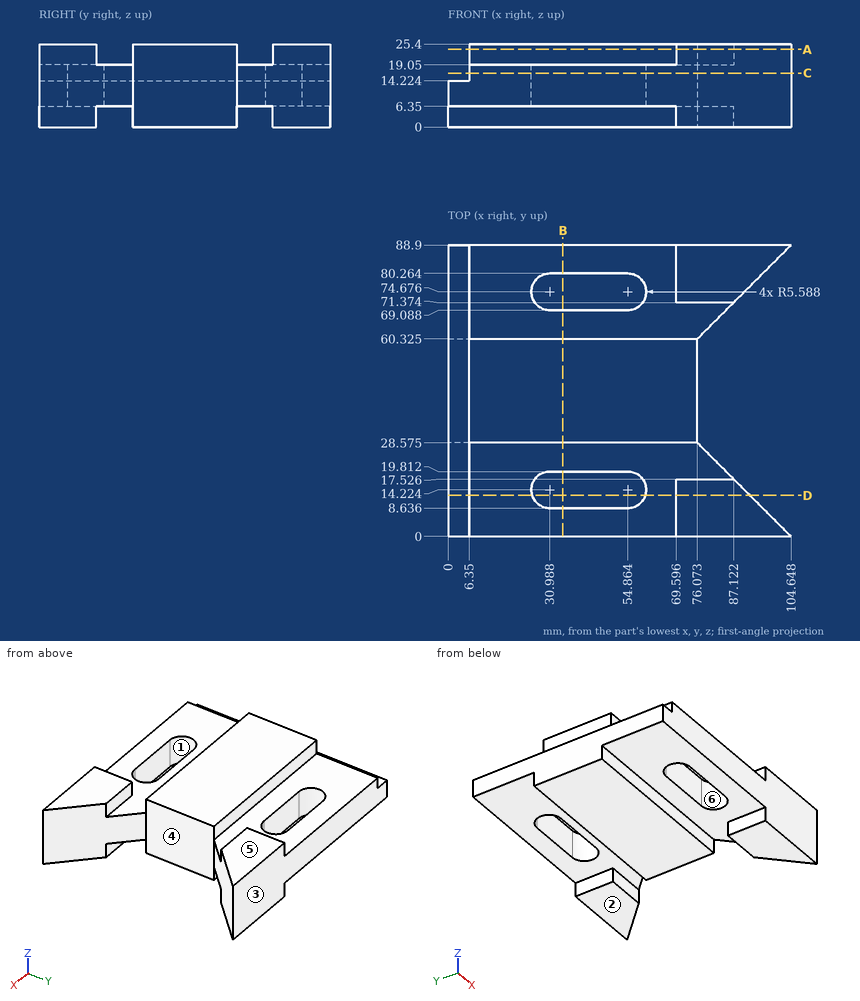
Check sheet for the drawn part. Datum: minimum x, y, z corner. Units: mm. A direction names the side the tool comes from. Round coordinates to 2 decimals unless told otherwise and drop trailing zeros. Loops run counter-clockwise (first coordinate to the right, second up) from the corner with the lowest first, then second, coordinate; pieces in that order, holes last. Notation, with made-up numbers: (-32.75, -36.5) - (-20.75, -36.5) arc R20 ccw to (-20.75, 2.5) - close; hole circle Ø9 at (70.25, 48.25). An arc over 180 degrees is marked (long way). Write item = value, one per line. Start each with the question number.
1. Section check D-D on y = 12.5. Enter the section's corners in (x, z).
2. Section check B-B on x = 35. Enter the section's corners in (y, z) (3 decimals), then the cut area to 3 significant figures.
3. Section check C-C on z = 16.5. Enter the section's corners in (x, y) (3 decimals), then the cut area to 3 significant figures.
4. Set-up check for the marked faces 4, 5 and 6: record each of +Z, -Z, +X, -X, +Y, -Y from which the full face is reachable in a straight line by a thin tool's end or side.
5. Mould release check, pull along Y, two halves, no side actions. Record for the marked faces 1, 2 and 3: released by +Y, released by -Y, zero draft, split by the parting line, or undercut.
6. Section check A-A on z = 23.75. Enter the section's corners in (x, y) (3 decimals).
7. Depth check by flat-ended pin: pin 1 (5 mm diameter, centred on x = 56, y = 71, fed in from -Z); pin 2 (3 mm diameter, centred on x = 75.5, y = 65, fed in from +Z); pin 3 (1.9 mm diameter, centred on x = 75.5, z = 4, fed in from -Y); pin 4 (3.5 mm diameter, centred on y = 44, z = 17, fed in from -X). Enter the tip coordinate at first touch or a pass-through.
8. Thickness scan on line 1 (Y direction, x = 35.5, z = 8.25); line 2 (Y direction, x = 73.5, z = 21.5) (3 decimals); line 3 (Z direction, x = 34.5, y = 85). Record the ranges inside material, lowest first.
Working result:
q1.outline = (0, 6.35) - (25.67, 6.35) - (25.67, 19.05) - (6.35, 19.05) - (6.35, 14.22) - (0, 14.22) - close; (60.18, 6.35) - (69.6, 6.35) - (69.6, 0) - (92.15, 0) - (92.15, 25.4) - (69.6, 25.4) - (69.6, 19.05) - (60.18, 19.05) - close
q2.outline = (0, 6.35) - (8.636, 6.35) - (8.636, 19.05) - (0, 19.05) - close; (19.812, 6.35) - (28.575, 6.35) - (28.575, 0) - (60.325, 0) - (60.325, 6.35) - (69.088, 6.35) - (69.088, 19.05) - (60.325, 19.05) - (60.325, 25.4) - (28.575, 25.4) - (28.575, 19.05) - (19.812, 19.05) - close; (80.264, 6.35) - (88.9, 6.35) - (88.9, 19.05) - (80.264, 19.05) - close
q2.area = 1,250 mm^2
q3.outline = (6.35, 0) - (104.648, 0) - (76.073, 28.575) - (76.073, 60.325) - (104.648, 88.9) - (6.35, 88.9) - close; hole (30.988, 8.636) - (54.864, 8.636) arc R5.588 ccw to (54.864, 19.812) - (30.988, 19.812) arc R5.588 ccw to start; hole (30.988, 69.088) - (54.864, 69.088) arc R5.588 ccw to (54.864, 80.264) - (30.988, 80.264) arc R5.588 ccw to start
q3.area = 6,290 mm^2
q4.face_4 = +Z, -Z, +X
q4.face_5 = +Z, +X, -X, +Y, -Y
q4.face_6 = +Z, -Z
q5.face_1 = undercut
q5.face_2 = zero draft
q5.face_3 = released by +Y
q6.outline = (6.35, 28.575) - (76.073, 28.575) - (76.073, 60.325) - (6.35, 60.325) - close; (69.596, 0) - (104.648, 0) - (87.122, 17.526) - (69.596, 17.526) - close; (69.596, 71.374) - (87.122, 71.374) - (104.648, 88.9) - (69.596, 88.9) - close
q7.pin_1 = 6.35
q7.pin_2 = 19.05
q7.pin_3 = 0
q7.pin_4 = 6.35
q8.line_1 = 0 to 8.64, 19.81 to 69.09, 80.26 to 88.9
q8.line_2 = 0 to 17.526, 28.575 to 60.325, 71.374 to 88.9
q8.line_3 = 6.35 to 19.05
